Source: three-view drawing plus pictorial views. Frame: mm from the lowest corner of the part. A direction names the side the tool comes from. Give positions to 0.01 mm unless a question says otherwise; leave off trailing zeros. Loops run counter-clockwise (first coordinate to the right, second up) from the corner with the lowest first, then second, coordinate; pieces in that order, holes last. Notation, with made-up numbers: (53.25, 74.5) - (108.25, 74.5) arc R22 cw to (108.25, 86.5) - close; hole circle Ø10 at (21.25, 59.5). An arc over 180 degrees is marked (long way). Put each result on its own line as item: value.
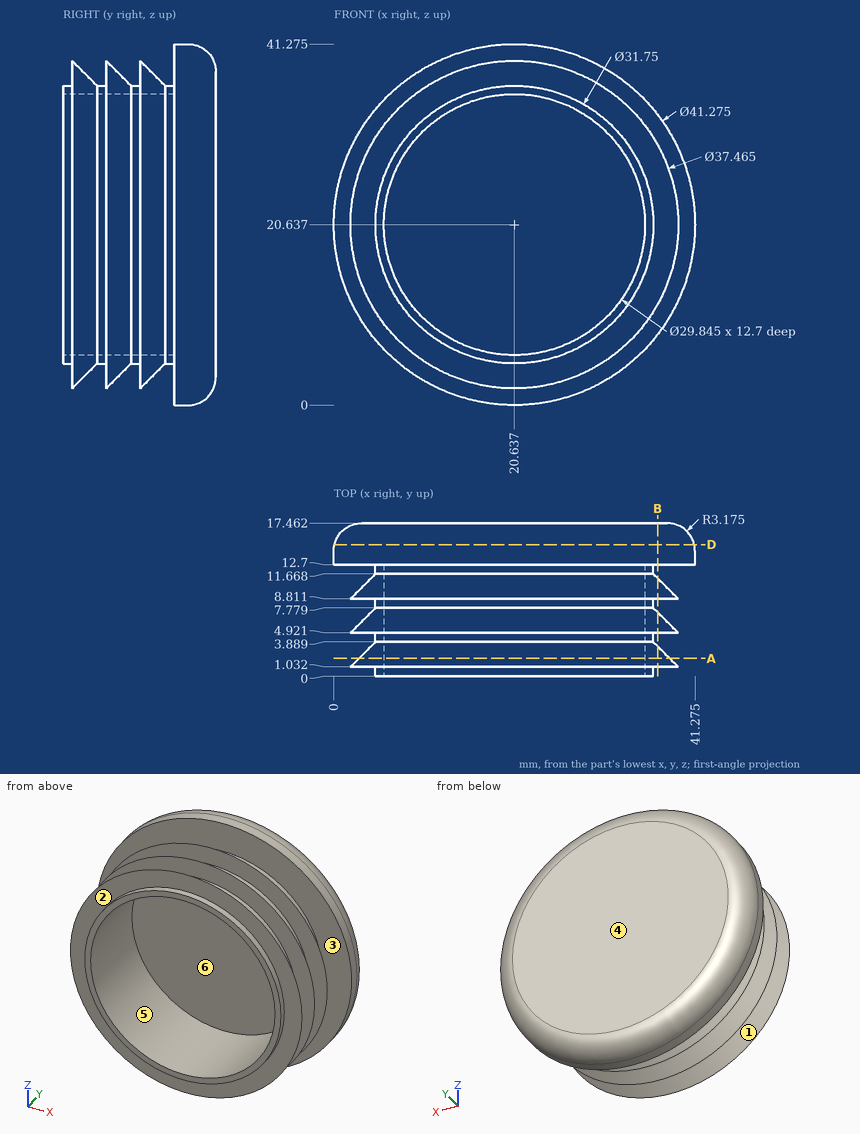
1) Mould query, pull axis Y, two halves, no side actions, for the marked faces 3, 4, 5 and 6. Classes: pulls with the +Y half, pulls with the -Y half, needs draft (parallel to the pull), parting line crosses it, or undercut.
Check result:
face 3: undercut
face 4: pulls with the +Y half
face 5: needs draft
face 6: pulls with the -Y half
2) Section query B-B, the plane x = 37. State how many separate pieces and enclosed holes the cut face has.
Check result:
separate pieces: 4
enclosed holes: 0
3) Pin query (flat end, axial travel): P1, Ø1, axis at y = 14.5, z = 8.5, coming from the -X side; P2, Ø18.5, axis at x = 11.5, z = 14, coming from the -Y side; P3, Ø1.5, axis at x = 25.5, y = 9.5, coming from the -Z side; P4, Ø1.5, axis at x = 31, z = 36.5, coming from the +Y side. Return the tip coordinate at first contact, or that it passes through.
Check result:
P1: x = 3.6
P2: y = 0
P3: z = 2.47
P4: y = 17.38
4) Section query A-A, the plane y = 2. Output: boundary loops of the cut face in (x, z) (1 decimal).
Check result:
outline: circle Ø35.5 at (20.6, 20.6); hole circle Ø29.8 at (20.6, 20.6)
5) Access query for the marked faces 1 and 2. Directions: +Z, -Z, +X, -X, +Y, -Y. A direction counts if a zero-diameter tool reaches every point of the face in a straight line with its end or side. Return the directions, or none.
Check result:
face 1: none
face 2: -Y
6) Material intervals for line 1 along Z through (x, y) = (16, 7.5) (1 decimal); line 2 along Z through (x, y) = (11.5, 7) (1 decimal); line 3 along Y through (x, z) = (36.5, 28) (1 decimal), sorted ascending. Write a range as [from, to].
Check result:
line 1: [5.2, 6.5], [34.8, 36.1]
line 2: [6.7, 8.8], [32.4, 34.6]
line 3: [1, 2.3], [4.9, 6.2], [8.8, 10.1], [12.7, 17.5]
7) Section query D-D, the plane y = 15. Output: boundary loops of the cut face in (x, z) (1 decimal), plus the area to 3 significant figures.
Check result:
outline: circle Ø41.1 at (20.6, 20.6)
area: 1,330 mm²
